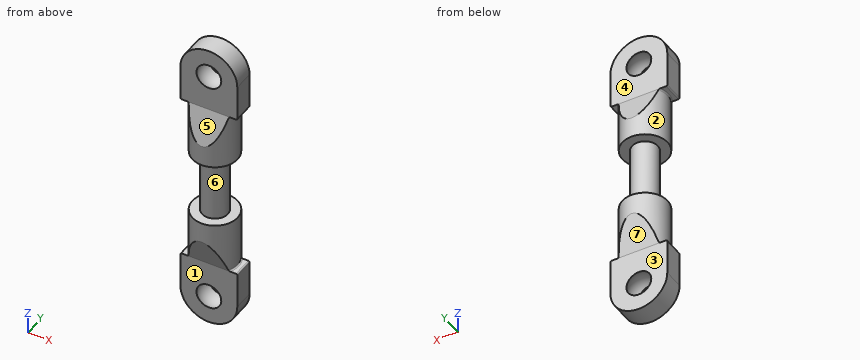
from build123d import *

# Parameters (mm, degrees)
SKETCH1_R                  = 2
SCREW_SECTION_DEPTH        = 5
SKETCH2_R                  = 3.5
BAR_SECTION_DEPTH          = 8.2
MOUNT_SECTION_DEPTH        = 1.6
BAR_TAPER_DEPTH            = 5.4
MOUNT_FILLET_R             = 0.2
MOUNT_FILLET_OF_MIRROR_2_R = 0.2


with BuildPart() as part:
    # Sketch1 → Screw Section (new body)
    with BuildSketch(Plane.XY):
        Circle(SKETCH1_R)
    screw_section = extrude(amount=SCREW_SECTION_DEPTH)

    # Sketch2 → Bar Section (add)
    with BuildSketch(Plane.XY.offset(5)):
        Circle(SKETCH2_R)
    bar_section = extrude(amount=BAR_SECTION_DEPTH)

    # Sketch3 → Mount Section (add, symmetric)
    with BuildSketch(Plane(origin=(0, 0, 0), x_dir=(1, 0, 0), z_dir=(0, 1, 0))):
        with BuildLine():
            Line((4.4, -13.2), (-4.4, -13.2))
            Line((-4.4, -13.2), (-4.4, -18.8))
            ThreePointArc((-4.4, -18.8), (0, -23.2), (4.4, -18.8))
            Line((4.4, -18.8), (4.4, -13.2))
        make_face()
    mount_section = extrude(amount=MOUNT_SECTION_DEPTH, both=True)

    # Sketch4 → Bar Taper (cut, symmetric)
    with BuildSketch(Plane(origin=(0, 0, 0), x_dir=(0, 0, -1), z_dir=(1, 0, 0))):
        Polygon((-8.2, -3.5), (-13.2, -1.6), (-13.2, -3.5), align=None)
        Polygon((-8.2, 3.5), (-13.2, 1.6), (-13.2, 3.5), align=None)
    bar_taper = extrude(amount=BAR_TAPER_DEPTH, both=True, mode=Mode.SUBTRACT)

    # Mount Fillet
    mount_fillet_edges = [part.edges().sort_by_distance(p)[0] for p in [
        (-4.4, 0, 13.2),
        (3.401842713, -0.823083322, 13.2),
        (-3.5, 0, 13.2),
        (4.4, 0, 13.2),
    ]]
    fillet(mount_fillet_edges, radius=MOUNT_FILLET_R)

    # Sketch6 → Ball Hole (revolve, cut)
    with BuildSketch(Plane(origin=(0, 0, 0), x_dir=(0, 0, -1), z_dir=(1, 0, 0))):
        with BuildLine():
            Line((-20.720937271, -1.6), (-18.8, -1.6))
            Line((-18.8, -1.6), (-18.8, 1.6))
            Line((-18.8, 1.6), (-20.720937271, 1.6))
            ThreePointArc((-20.720937271, 1.6), (-21.3, 0), (-20.720937271, -1.6))
        make_face()
    ball_hole = revolve(axis=Axis((0, -1.6, 18.8), (0, 1, 0)), mode=Mode.SUBTRACT)

    # Mirror 2: Screw Section, Bar Section, Mount Section, Bar Taper, Ball Hole across Front Plane
    add(screw_section.mirror(Plane.XY))
    add(bar_section.mirror(Plane.XY))
    add(mount_section.mirror(Plane.XY))
    add(bar_taper.mirror(Plane.XY), mode=Mode.SUBTRACT)
    add(ball_hole.mirror(Plane.XY), mode=Mode.SUBTRACT)

    # Mount Fillet of Mirror 2
    mount_fillet_of_mirror_2_edges = [part.edges().sort_by_distance(p)[0] for p in [
        (-4.4, 0, -13.2),
        (3.401842713, -0.823083322, -13.2),
        (-3.5, 0, -13.2),
        (4.4, 0, -13.2),
    ]]
    fillet(mount_fillet_of_mirror_2_edges, radius=MOUNT_FILLET_OF_MIRROR_2_R)


solid = part.part
Read the model definition and answer for the solid it produces. Units are mm, in the model's axes. Face numbers are marked on the shaded views. A direction names the side the tool comes from. Give positions to 0.01 mm unless a question says otherwise; leave off trailing zeros. Write each loop counter-clockwise with the first axis right and the second up, starting at its lowest first coordinate (ties: lowest second). Pieces come first, ordered by that corner, then holes. Notation, with made-up numbers: (54.5, -17) - (86.5, -17) arc R26 ccw to (86.5, 12) - close; hole circle Ø2 at (-4.5, -30.75). An arc over 180 degrees is marked (long way). Answer in a Markdown table with one row per item. Add a question column.
Item 1: Section B-B, the plane x = -1.25 is taken. Write down the section's boundary in (y, z), and give its area (3 significant figures).
Item 2: Section A-A, the plane z = 17.5 is taken. Write down the section's boundary in (x, y), and give its area (3 significant figures).
Item 3: A tool of negligible diameter and unlimited length cuts with its end or side. For the marked faces 1, 2, 3 and 4, from which of +Z, -Z, +X, -X, +Y, -Y can it reach the whole face along a straight path? Write none if from no direction.
Item 4: Determine the mould class of the marked faces 5, 6 and 7 for opening direction Z: pulls with the +Z half, pulls with the -Z half, needs draft (parallel to the pull), parting line crosses it, or undercut.
Item 5: Flat-ended cylindrical pins translate along their axes: P1, Ø4.5, axis at x = 2, z = 18.5, coming from the +Y side; P2, Ø0.7, axis at x = 3.5, y = 0.5, coming from the -Z side; P3, Ø1, axis at x = 2, y = -1.5, coming from the +Z side. Find the tip coordinate at first contact, or state that the pin passes through.
Item 6: Section C-C, the plane y = 3 is taken. Write down the section's boundary in (x, z).
Item 7: Find the intervals of material crossed by L1, parallel to Z at x = 1, y = 1.5; L2, parallel to Z at x = 2.75, y = 0.5; L3, parallel to Z at x = -4, y = 1.5, in increasing order.
Recorded:
| question | item | result |
|---|---|---|
| 1 | outline | (-3.27, -8.81) - (-1.6, -13.2) - (-1.6, -17.34) arc R2.17 cw to (1.6, -17.34) - (1.6, -13.2) - (3.27, -8.81) - (3.27, -5) - (1.56, -5) - (1.56, 5) - (3.27, 5) - (3.27, 8.81) - (1.6, 13.2) - (1.6, 17.34) arc R2.17 cw to (-1.6, 17.34) - (-1.6, 13.2) - (-3.27, 8.81) - (-3.27, 5) - (-1.56, 5) - (-1.56, -5) - (-3.27, -5) - close; (-1.6, -23.02) - (1.6, -23.02) - (1.6, -20.26) arc R2.17 cw to (-1.6, -20.26) - close; (-1.6, 20.26) arc R2.17 cw to (1.6, 20.26) - (1.6, 23.02) - (-1.6, 23.02) - close |
| 1 | area | 162 mm2 |
| 2 | outline | (-4.4, -1.6) - (-1.41, -1.6) arc R2.14 cw to (-1.41, 1.6) - (-4.4, 1.6) - close; (1.41, -1.6) - (4.4, -1.6) - (4.4, 1.6) - (1.41, 1.6) arc R2.14 cw to start |
| 2 | area | 15.9 mm2 |
| 3 | face 1 | -Z, +X, -X, -Y |
| 3 | face 2 | none |
| 3 | face 3 | -Z, +X, -X, +Y |
| 3 | face 4 | +Z, +X, -X, +Y |
| 4 | face 5 | pulls with the +Z half |
| 4 | face 6 | undercut |
| 4 | face 7 | pulls with the -Z half |
| 5 | P1 | stops at y = 1.6 |
| 5 | P2 | stops at z = -21.87 |
| 5 | P3 | stops at z = 22.94 |
| 6 | outline | (-1.8, -9.52) - (1.8, -9.52) - (1.8, -5) - (-1.8, -5) - close; (-1.8, 5) - (1.8, 5) - (1.8, 9.52) - (-1.8, 9.52) - close |
| 7 | L1 | z = -23.08 to -20.53, -17.07 to 17.07, 20.53 to 23.08 |
| 7 | L2 | z = -22.23 to -5, 5 to 22.23 |
| 7 | L3 | z = -20.63 to -13.2, 13.2 to 20.63 |
